Job drawing, mm, ordinate dimensions from the low corner. One solid piece. Round coordinates to 2 decimals unless told otherwise and drop trailing zeros. Loops run counter-clockwise (first coordinate to the right, second up) from the corner with the lowest first, then second, coordinate; pieces in that order, holes last.
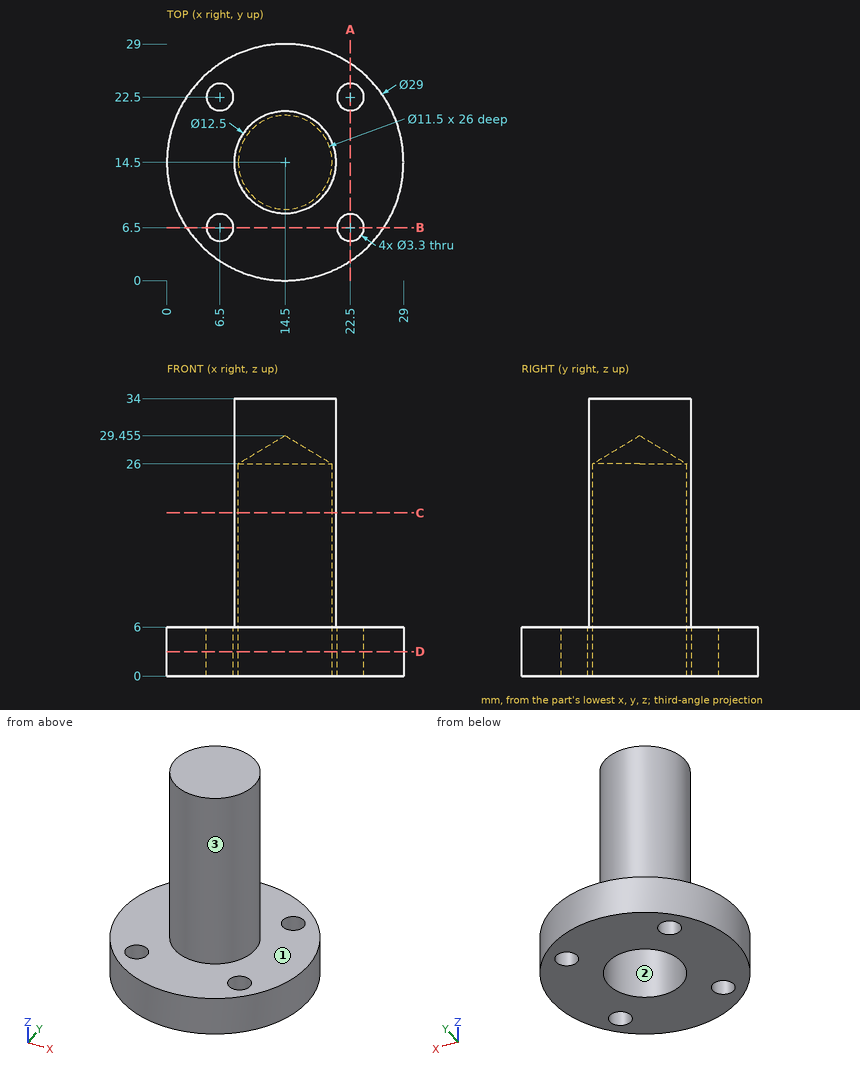
Item 1: Cut at C-C, the plane z = 20. Give the cut face in (x, y).
Answers follow:
outline: circle Ø12.5 at (14.5, 14.5); hole circle Ø11.5 at (14.5, 14.5)
Item 2: Cut at A-A, the plane x = 22.5. Give the cut face in (y, z), plus the area to 3 significant figures.
Answers follow:
outline: (2.41, 0) - (4.85, 0) - (4.85, 6) - (2.41, 6) - close; (8.15, 0) - (20.85, 0) - (20.85, 6) - (8.15, 6) - close; (24.15, 0) - (26.59, 0) - (26.59, 6) - (24.15, 6) - close
area: 106 mm2
Item 3: Probe line 1 (Y direction, x = 14.5, z = 5.75); line 2 (X direction, y = 22.5, z = 1.35). List the from-to ranges inside material, lowest first.
Answers follow:
line 1: y = 0 to 8.75, 20.25 to 29
line 2: x = 2.41 to 4.85, 8.15 to 20.85, 24.15 to 26.59
Item 4: Two-plate mould, pull along X, no slides. Class the marked faces 1, 2 and 3: released by +X, released by -X, zero draft, split by the parting line, or undercut.
Answers follow:
face 1: zero draft
face 2: undercut
face 3: split by the parting line
Item 5: Flat gauge pins, fed straight in: P1, Ø6, axis at x = 10.5, z = 27, coming from the +Y side; P2, Ø5, axis at y = 22.5, z = 18, coming from the +X side; P3, Ø8, axis at x = 8.5, z = 6, coming from the +Y side. Where does each tip first touch, or does it go through?
Answers follow:
P1: stops at y = 20.67
P2: stops at x = 17.47
P3: stops at y = 28.86
Item 6: Cut at D-D, the plane z = 3. Give the cut face in (x, y), plus the area to 3 significant figures.
Answers follow:
outline: circle Ø29 at (14.5, 14.5); hole circle Ø3.3 at (6.5, 6.5); hole circle Ø3.3 at (6.5, 22.5); hole circle Ø11.5 at (14.5, 14.5); hole circle Ø3.3 at (22.5, 6.5); hole circle Ø3.3 at (22.5, 22.5)
area: 522 mm2
